```python
from build123d import *

# Parameters (mm, degrees)
F0_W     = 18.1666671749
F0_H     = 1
F0_W_2   = 29.6666571914
F0_H_2   = 15.3333324809
F0_W_3   = 18.0000001967
F1_DEPTH = 25
F2_R     = 5
F3_R     = 5
F4_R     = 5
F5_R     = 5
F6_R     = 5
F7_R     = 5
F8_R     = 5
F9_R     = 5
F10_R    = 5
F11_R    = 5
F13_D    = 8
F15_D    = 8


with BuildPart() as f1:
    # F0 (on Front) → F1 (new body)
    with BuildSketch(Plane.XZ):
        with Locations((25.416871541, 26.1666653552)):
            Rectangle(F0_W, F0_H)
        Polygon((34.5002051284, 26.6666653552), (51.3333348415, 26.6666653552), (51.3333348415, 40), (0, 40), (0, 26.6666653552), (16.3335379536, 26.6666653552), align=None)
        Polygon((51.3333348415, 11.3333328743), (51.3333348415, 0), (62.3333337596, 0), (62.3333337596, 11.3333328743), (62.3333337596, 26.6666653552), (62.3333337596, 40), (51.3333348415, 40), (51.3333348415, 26.6666653552), align=None)
        with Locations((77.1666623552, 18.9999991148)):
            Rectangle(F0_W_2, F0_H_2)
        Polygon((0, 11.3333328743), (0, 0), (51.3333348415, 0), (51.3333348415, 11.3333328743), (34.5002051284, 11.3333328743), (16.5002049317, 11.3333328743), align=None)
        with Locations((25.5002050301, 11.8333328743)):
            Rectangle(F0_W_3, F0_H)
    extrude(amount=F1_DEPTH)

    # F2
    f2_edges = [f1.edges().sort_by_distance(p)[0] for p in [
        (62.333334, -12.5, 40),
    ]]
    fillet(f2_edges, radius=F2_R)

    # F3
    f3_edges = [f1.edges().sort_by_distance(p)[0] for p in [
        (62.333334, -12.5, 26.666665),
    ]]
    fillet(f3_edges, radius=F3_R)

    # F4
    f4_edges = [f1.edges().sort_by_distance(p)[0] for p in [
        (91.999991, -12.5, 26.666665),
    ]]
    fillet(f4_edges, radius=F4_R)

    # F5
    f5_edges = [f1.edges().sort_by_distance(p)[0] for p in [
        (0, -12.5, 40),
    ]]
    fillet(f5_edges, radius=F5_R)

    # F6
    f6_edges = [f1.edges().sort_by_distance(p)[0] for p in [
        (0, -12.5, 26.666665),
    ]]
    fillet(f6_edges, radius=F6_R)

    # F7
    f7_edges = [f1.edges().sort_by_distance(p)[0] for p in [
        (0, -12.5, 11.333333),
    ]]
    fillet(f7_edges, radius=F7_R)

    # F8
    f8_edges = [f1.edges().sort_by_distance(p)[0] for p in [
        (0, -12.5, 0),
    ]]
    fillet(f8_edges, radius=F8_R)

    # F9
    f9_edges = [f1.edges().sort_by_distance(p)[0] for p in [
        (62.333334, -12.5, 0),
    ]]
    fillet(f9_edges, radius=F9_R)

    # F10
    f10_edges = [f1.edges().sort_by_distance(p)[0] for p in [
        (62.333334, -12.5, 11.333333),
    ]]
    fillet(f10_edges, radius=F10_R)

    # F11
    f11_edges = [f1.edges().sort_by_distance(p)[0] for p in [
        (91.999991, -12.5, 11.333333),
    ]]
    fillet(f11_edges, radius=F11_R)

    # F13 (through all)
    with Locations(Plane.XY.offset(40)):
        with Locations((22.7013193071, -12.9694240168)):
            Hole(F13_D / 2)

    # F15 (through all)
    with Locations(Plane(origin=(0, 0, 11.3333328743), x_dir=(1, 0, 0), z_dir=(0, 0, -1))):
        with Locations((79.9189954996, 12.5)):
            Hole(F15_D / 2)


solid = f1.part
```
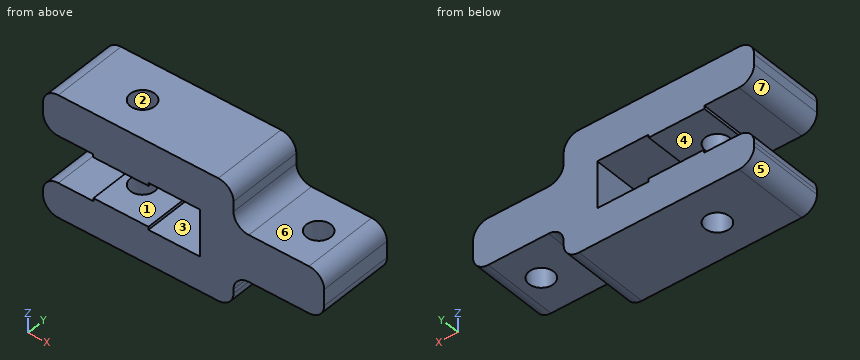
Source: CAD feature listing. Evaluate the final solid. Frame: model axes, mm. Face numbers are marked on the shaded views. A direction names the side the tool comes from. Round coordinates to 2 decimals unless told otherwise and drop trailing zeros. Loops run counter-clockwise (first coordinate to the right, second up) from the corner with the lowest first, then second, coordinate; pieces in that order, holes last.
1. Section query B-B on x = 78.5. Output: boundary loops of the cut face in (y, z).
2. Mould query, pull axis Z, two halves, no side actions, for the marked faces 4, 5, 6 and 7. Classes: released by +Z, released by -Z, zero draft, split by the parting line, or undercut.
3. Contact query for flat-ended pins moving along their axis: pin 1 (1.1 mm diameter, centred on y = -12.5, z = 12, fed in from -X); pin 2 (5 mm diameter, centred on y = -12, z = 27, fed in from -X); pin 3 (8 mm diameter, centred on y = -14.5, z = 31.5, fed in from +X); pin 4 (5 mm diameter, centred on x = 22.7, y = -12.97, fed in from +Z). Output: stop coordinate, or through.
4. Access query for the marked faces 1, 2 and 3. Directions: +Z, -Z, +X, -X, +Y, -Y. A direction counts if a zero-diameter tool reaches every point of the face in a straight line with its end or side. Return the directions, or none.
5. Ray query, L1, parallel to Z at x = 14.5, y = -16; L2, parallel to Z at x = 28, y = -22; L3, parallel to Z at x = 81, y = -5. Return the intervals inside material, ascending.
6. Section query D-D on z = 22.5. Output: boundary loops of the cut face in (x, y).
7. Section query A-A on x = 20. Output: boundary loops of the cut face in (y, z), and give its area (3 significant figures).
Answers below:
1. outline: (-25, 11.33) - (-16.24, 11.33) - (-16.24, 26.67) - (-25, 26.67) - close; (-8.76, 11.33) - (0, 11.33) - (0, 26.67) - (-8.76, 26.67) - close
2. face 4: undercut
2. face 5: released by -Z
2. face 6: released by +Z
2. face 7: undercut
3. pin 1: stops at x = 16.5
3. pin 2: stops at x = 0.49
3. pin 3: stops at x = 64.57
3. pin 4: passes through
4. face 1: -X, +Y, -Y
4. face 2: +Z, -Z
4. face 3: +Y, -Y
5. L1: z = 0 to 11.33, 26.67 to 40
5. L2: z = 0 to 12.33, 25.67 to 40
5. L3: z = 11.33 to 26.67
6. outline: (51.33, -25) - (91.93, -25) - (91.93, 0) - (51.33, 0) - close; hole circle Ø8 at (79.92, -12.5)
7. outline: (-25, 0) - (-15.92, 0) - (-15.92, 12.33) - (-25, 12.33) - close; (-25, 25.67) - (-15.92, 25.67) - (-15.92, 40) - (-25, 40) - close; (-10.02, 0) - (0, 0) - (0, 12.33) - (-10.02, 12.33) - close; (-10.02, 25.67) - (0, 25.67) - (0, 40) - (-10.02, 40) - close
7. area: 509 mm2
